Work out the finished part from the listing and answer in its coordinate system (mm). Give positions to 0.01 mm unless a question says otherwise; leave off trailing zeros. Loops run counter-clockwise (first coordinate to the right, second up) from the corner with the lowest first, then second, coordinate; pieces in that order, holes last.
```python
from build123d import *

# Parameters (mm, degrees)
F1_DEPTH = 1
F2_W     = 8
F2_H     = 8
F3_DEPTH = 1


# Not quite as in the source:
# - a feature names something its author has since deleted; it is built from what else it names


with BuildPart() as f1:
    # F0 (on Top) → F1 (new body)
    with BuildSketch(Plane.XY):
        Polygon((0, 20), (-50, 0), (0, 0), align=None)
    extrude(amount=F1_DEPTH)

    # F2 (on face) → F3 (join)
    with BuildSketch(Plane.XY.offset(1)):
        Polygon((-19, 11.3229670386), (-19, 11), (-11, 11), (-11, 14.5229670386), align=None)
        Polygon((-29, 7.3229670386), (-29, 1), (-21, 1), (-21, 9), (-24.8074175964, 9), align=None)
        Polygon((-39, 3.3229670386), (-39, 1), (-31, 1), (-31, 6.5229670386), align=None)
        Polygon((-9, 15.3229670386), (-9, 11), (-1, 11), (-1, 18.5229670386), align=None)
        with Locations((-5, 5)):
            Rectangle(F2_W, F2_H)
        with Locations((-15, 5)):
            Rectangle(F2_W, F2_H)
        Polygon((-41, 2.5229670386), (-44.8074175964, 1), (-41, 1), align=None)
    extrude(amount=F3_DEPTH)


solid = f1.part
```
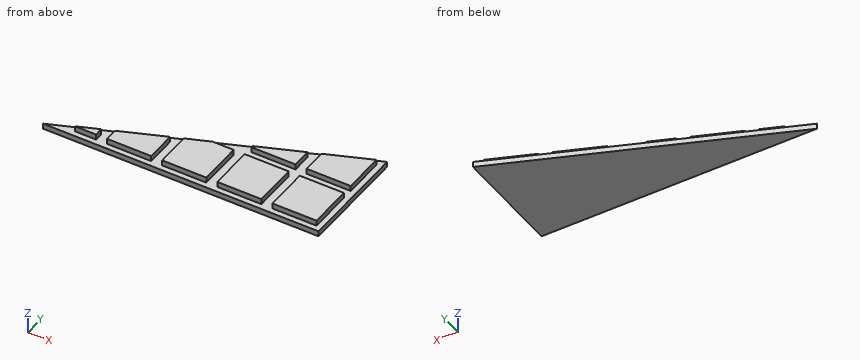
Q1. Section D-D on x = -4 is taken. Give the vertices of the cut face in (y, z).
Q2. Section A-A on z = 1.5 is taken. Give the vertices of the cut face in (x, y), plus the area to 3 significant figures.
Q3. Section B-B on x = -36 is taken. Give the vertices of the cut face in (y, z).
Q4. Section C-C on y = 10 is taken. Give the vertices of the cut face in (x, z).
Q5. Consider line 1 along X through (y, z) = (7, 1.25); line 2 along X through (y, z) = (11.25, 1.3); line 3 along X through (y, z) = (15.25, 1.15). Determine where each line is inside the solid, lowest interval first.
Q6. Given pin 1 (0.8 mm diameter, centred on x = -14.5, z = 1.5, fed in from -Y); pin 2 (0.8 mm diameter, centred on x = -23, z = 1.5, fed in from +Y); pin 3 (0.8 mm diameter, centred on y = 2.5, z = 1.5, fed in from -X), each flat-ended and moving along its own axis, determine where each tip first touches the part or whether it passes through.
Check result:
1. outline: (0, 0) - (18.4, 0) - (18.4, 1) - (17.32, 1) - (17.32, 2) - (11, 2) - (11, 1) - (9, 1) - (9, 2) - (1, 2) - (1, 1) - (0, 1) - close
2. outline: (-44.81, 1) - (-41, 1) - (-41, 2.52) - close; (-39, 1) - (-31, 1) - (-31, 6.52) - (-39, 3.32) - close; (-29, 1) - (-21, 1) - (-21, 9) - (-24.81, 9) - (-29, 7.32) - close; (-19, 1) - (-11, 1) - (-11, 9) - (-19, 9) - close; (-19, 11) - (-11, 11) - (-11, 14.52) - (-19, 11.32) - close; (-9, 1) - (-1, 1) - (-1, 9) - (-9, 9) - close; (-9, 11) - (-1, 11) - (-1, 18.52) - (-9, 15.32) - close
2. area: 286 mm2
3. outline: (0, 0) - (5.6, 0) - (5.6, 1) - (4.52, 1) - (4.52, 2) - (1, 2) - (1, 1) - (0, 1) - close
4. outline: (-25, 0) - (0, 0) - (0, 1) - (-25, 1) - close
5. line 1: x = -29 to -21, -19 to -11, -9 to -1
5. line 2: x = -19 to -11, -9 to -1
5. line 3: x = -9 to -1
6. pin 1: stops at y = 1
6. pin 2: stops at y = 9
6. pin 3: stops at x = -42.06
